For this review, take the finished solid that the model builds, in its own axes (mm). Give positions to 0.01 mm unless a question says otherwise; leave off trailing zeros. Order: outer loops, then holes, each group sorted by start corner. A loop starts at its lowest first (then second) coordinate and runs counter-clockwise, first axis right, second up. Notation, with made-up numbers: (-15, 64) - (30, 64) arc R34 ccw to (30, 100) - close; hole circle Ø3 at (21, 56). An arc over 180 degrees is marked (long way). One line per item, written item: value.
```python
from build123d import *

# Parameters (mm, degrees)
F0_W     = 25
F0_H     = 4.875
F0_H_2   = 10.25
F1_DEPTH = 3
F2_R     = 1
F3_R     = 2
F4_DEPTH = 68


with BuildPart() as f1:
    # F0 (on Top) → F1 (new body)
    with BuildSketch(Plane.XY):
        with Locations((0, 7.5625)):
            Rectangle(F0_W, F0_H)
        with Locations((0, -7.5625)):
            Rectangle(F0_W, F0_H)
        Rectangle(F0_W, F0_H_2)
    extrude(amount=F1_DEPTH)

    # F2
    f2_edges = [f1.edges().sort_by_distance(p)[0] for p in [
        (0, -10, 3),
        (12.5, 0, 3),
        (0, 10, 3),
        (-12.5, 0, 3),
        (12.5, -10, 1.5),
        (-12.5, -10, 1.5),
        (-12.5, 10, 1.5),
        (12.5, 10, 1.5),
    ]]
    fillet(f2_edges, radius=F2_R)

    # F3 (on face) → F4 (cut)
    with BuildSketch(Plane.XY):
        with BuildLine():
            ThreePointArc((-9, -5), (-10.414214, -8.414214), (-7, -7))
            ThreePointArc((-7, -7), (-7.585786, -5.585786), (-9, -5))
        make_face()
        with Locations((9, -7)):
            Circle(F3_R)
        with Locations((9, 7)):
            Circle(F3_R)
        with Locations((-9, 7)):
            Circle(F3_R)
    extrude(amount=F4_DEPTH, mode=Mode.SUBTRACT)


solid = f1.part
```
(1) Take a section at B-B (x = 10). Write out the cut boundary in (y, z).
Answers below:
outline: (-10, 0) - (-8.73, 0) - (-8.73, 3) - (-9, 3) arc R1 ccw to (-10, 2) - close; (-5.27, 0) - (5.27, 0) - (5.27, 3) - (-5.27, 3) - close; (8.73, 0) - (10, 0) - (10, 2) arc R1 ccw to (9, 3) - (8.73, 3) - close
(2) Take a section at A-A (y = 7). Write out the cut boundary in (x, z).
Answers below:
outline: (-12.5, 0) - (-11, 0) - (-11, 3) - (-11.5, 3) arc R1 ccw to (-12.5, 2) - close; (-7, 0) - (7, 0) - (7, 3) - (-7, 3) - close; (11, 0) - (12.5, 0) - (12.5, 2) arc R1 ccw to (11.5, 3) - (11, 3) - close
(3) Wall thickness on line 1 (Y direction, x = 9, z = 1.7); line 2 (X direction, y = 7, z = 2); line 3 (X direction, y = -8.25, z = 0.4): over which ranges is each line inside the solid? List them lowest first. Write a range as from..to.
Answers below:
line 1: y = -10..-9, -5..5, 9..10
line 2: x = -12.5..-11, -7..7, 11..12.5
line 3: x = -12.5..-10.56, -7.44..7.44, 10.56..12.5
(4) Draft analysis for pull direction X (two halves, no side actions). For faces 1 (the face through (0, 0, 3)), 2 (the face through (7, -7, 1)), 3 (the face through (12.215, 9.699, 1.014)), state which applies: pulls with the +X half, pulls with the -X half, needs draft (parallel to the pull), parting line crosses it, or undercut.
Answers below:
face 1: needs draft
face 2: undercut
face 3: pulls with the +X half
(5) Take a section at D-D (z = 1.45). Write out the cut boundary in (x, y), then the cut area to 3 significant figures.
Answers below:
outline: (-12.5, -9) arc R1 ccw to (-11.5, -10) - (11.5, -10) arc R1 ccw to (12.5, -9) - (12.5, 9) arc R1 ccw to (11.5, 10) - (-11.5, 10) arc R1 ccw to (-12.5, 9) - close; hole circle Ø4 at (-9, 7); hole (-9, -5) arc R2 ccw (long way) to (-7, -7) arc R2 ccw to start; hole circle Ø4 at (9, -7); hole circle Ø4 at (9, 7)
area: 449 mm^2
(6) Take a section at C-C (z = 2.6). Write out the cut boundary in (x, y).
Answers below:
outline: (-12.3, -9) arc R0.8 ccw to (-11.5, -9.8) - (11.5, -9.8) arc R0.8 ccw to (12.3, -9) - (12.3, 9) arc R0.8 ccw to (11.5, 9.8) - (-11.5, 9.8) arc R0.8 ccw to (-12.3, 9) - close; hole circle Ø4 at (-9, 7); hole (-9, -5) arc R2 ccw (long way) to (-7, -7) arc R2 ccw to start; hole circle Ø4 at (9, -7); hole circle Ø4 at (9, 7)
